from build123d import *

# Parameters (mm, degrees)
F0_W     = 4.2672
F0_H     = 5.842
F0_W_2   = 7.894506
F0_H_2   = 31.5722
F0_W_3   = 7.912528
F1_DEPTH = 4.3434


with BuildPart() as f1:
    # F0 (on Front) → F1 (new body)
    with BuildSketch(Plane.XZ):
        Polygon((38.080222, -15.7861), (38.080222, 15.7861), (-38.080222, 15.7861), (-38.080222, -15.7861), (-3.443861, -15.758646), (-3.443861, -8.138646), (3.414139, -8.138646), (3.414139, -15.758646), align=None)
        with Locations((-25.151622, -9.0043)):
            Rectangle(F0_W, F0_H, mode=Mode.SUBTRACT)
        with Locations((25.151622, -9.0043)):
            Rectangle(F0_W, F0_H, mode=Mode.SUBTRACT)
        with Locations((-25.151622, 9.0043)):
            Rectangle(F0_W, F0_H, mode=Mode.SUBTRACT)
        with Locations((25.151622, 9.0043)):
            Rectangle(F0_W, F0_H, mode=Mode.SUBTRACT)
        with Locations((42.027475, 0)):
            Rectangle(F0_W_2, F0_H_2)
        with Locations((-42.036486, 0)):
            Rectangle(F0_W_3, F0_H_2)
        with BuildLine():
            ThreePointArc((45.974728, -15.7861), (50.240287, 0), (45.974728, 15.7861))
            Line((45.974728, 15.7861), (45.974728, -15.7861))
        make_face()
        with BuildLine():
            Line((-45.99275, -15.7861), (-45.99275, 15.7861))
            ThreePointArc((-45.99275, 15.7861), (-50.259919, 0), (-45.99275, -15.7861))
        make_face()
    extrude(amount=F1_DEPTH)


solid = f1.part
Model file for the job. Use its own axes, mm. A direction names the side the tool comes from. Give positions to 0.01 mm unless a question says otherwise; leave off trailing zeros. Loops run counter-clockwise (first coordinate to the right, second up) from the corner with the lowest first, then second, coordinate; pieces in that order, holes last.
1) Saw through at C-C (z = -10). Write the cut outline in (x, y).
2) Saw through at B-B (y = -3.65). Write the cut outline in (x, z), plus the area to 3 significant figures.
3) Pull direction Z, two halves, no side cores. Call faces 1 (the flat face through (0, -2, -8.139)), 2 (the cylindrical face through (50.24, -2.14, -0.23)), 3 (the flat face through (25, -2, 11.925)): +Z half, -Z half, draft (parallel to the pull), parting line (faces both ways), or undercut.
4) Wall check: line 1 (X direction, y = -3.4, z = -8.5); line 2 (X direction, y = -0.25, z = -9); line 3 (X direction, y = -2.6, z = -7.5). Give the ranges that are in metal, low to high.
5) Saw through at A-A (z = 10). Write the cut outline in (x, y), plus the area to 3 significant figures.
6) Tool access for faces 4 (the flat face through (3.414, -2, -12)), 5 (the flat face through (-1, -4.343, 0)), 6 (the flat face through (-27.285, -2, 9)): list every direction of +Z, -Z, +X, -X, +Y, -Y with a clear straight run to the whole face (end or side of a thin tool).
7) Flat gauge pins, fed straight in: pin 1 Ø1.3 at (x, y) = (-25, -3) entering from -Z; pin 2 Ø1.3 at (y, z) = (-2, -8.5) entering from +X; pin 3 Ø1.3 at (y, z) = (-2, -11.5) entering from -X. Where does each tip first touch, or does it go through?
Answer block:
1. outline: (-48.62, -4.34) - (-27.29, -4.34) - (-27.29, 0) - (-48.62, 0) - close; (-23.02, -4.34) - (-3.44, -4.34) - (-3.44, 0) - (-23.02, 0) - close; (3.41, -4.34) - (23.02, -4.34) - (23.02, 0) - (3.41, 0) - close; (27.29, -4.34) - (48.6, -4.34) - (48.6, 0) - (27.29, 0) - close
2. outline: (-45.99, -15.79) - (-38.08, -15.79) - (-3.44, -15.76) - (-3.44, -8.14) - (3.41, -8.14) - (3.41, -15.76) - (38.08, -15.79) - (45.97, -15.79) arc R31.34 ccw to (45.97, 15.79) - (-45.99, 15.79) arc R31.33 ccw to start; hole (-27.29, -11.93) - (-23.02, -11.93) - (-23.02, -6.08) - (-27.29, -6.08) - close; hole (-27.29, 6.08) - (-23.02, 6.08) - (-23.02, 11.93) - (-27.29, 11.93) - close; hole (23.02, -11.93) - (27.29, -11.93) - (27.29, -6.08) - (23.02, -6.08) - close; hole (23.02, 6.08) - (27.29, 6.08) - (27.29, 11.93) - (23.02, 11.93) - close
2. area: 2,930 mm2
3. face 1: -Z half
3. face 2: parting line
3. face 3: undercut
4. line 1: x = -49.08 to -27.29, -23.02 to -3.44, 3.41 to 23.02, 27.29 to 49.07
4. line 2: x = -48.94 to -27.29, -23.02 to -3.44, 3.41 to 23.02, 27.29 to 48.92
4. line 3: x = -49.35 to -27.29, -23.02 to 23.02, 27.29 to 49.33
5. outline: (-48.62, -4.34) - (-27.29, -4.34) - (-27.29, 0) - (-48.62, 0) - close; (-23.02, -4.34) - (23.02, -4.34) - (23.02, 0) - (-23.02, 0) - close; (27.29, -4.34) - (48.6, -4.34) - (48.6, 0) - (27.29, 0) - close
5. area: 385 mm2
6. face 4: -Z, +Y, -Y
6. face 5: +Z, -Z, +X, -X, -Y
6. face 6: +Y, -Y
7. pin 1: stops at z = -15.78
7. pin 2: stops at x = 49.24
7. pin 3: stops at x = -48.32
